Autodesk Inventor part; units mm, degrees
ref_plane "Arbeitsebene1" through (14, 0, 0) normal (1, 0, 0) x (0, 1, 0)
ref_plane "XZ Plane" through (0, 0, 0) normal (0, 1, 0) x (-1, 0, 0)
ref_plane "XY Plane" through (0, 0, 0) normal (0, 0, 1) x (1, 0, 0)
sketch "Skizze1" plane through (0, 0, 0) normal (0, 0, 1) x (1, 0, 0)
  line L0 (0, 20) -> (28, 20)
  line L1 (28, 20) -> (28, 0)
  line L2 (28, 0) -> (0, 0)
  line L3 (0, 0) -> (0, 20)
  dimension "d0" = 28
  dimension "d1" = 20
extrude "Extrusion1" add sketch "Skizze1" along normal blind 3
sketch "Skizze2" plane through (0, 0, 3) normal (0, 0, 1) x (1, 0, 0)
  line L0 (0, 20) -> (0, 0)
  line L1 (0, 10) -> (28.5763, 10) construction
  line L2 (28, 0) -> (28, 20)
  point P0 (3, 17)
  point P1 (3, 3)
  point P2 (25, 17)
  point P3 (25, 3)
  dimension "d4" = 14
  dimension "d5" = 3
  dimension "d14" = 3
hole "Bohrung1" at (3, 17, 3) at (3, 3, 3) at (25, 3, 3) at (25, 17, 3) direction (0, 0, -1) diameter 1.4 end through all countersink diameter 3 countersink angle 90
ref_plane "Arbeitsebene1" through (14, 0, 0) normal (1, 0, 0) x (0, 1, 0)
properties part number "Zylinderkopf" material "Stahl, galvanisiert"
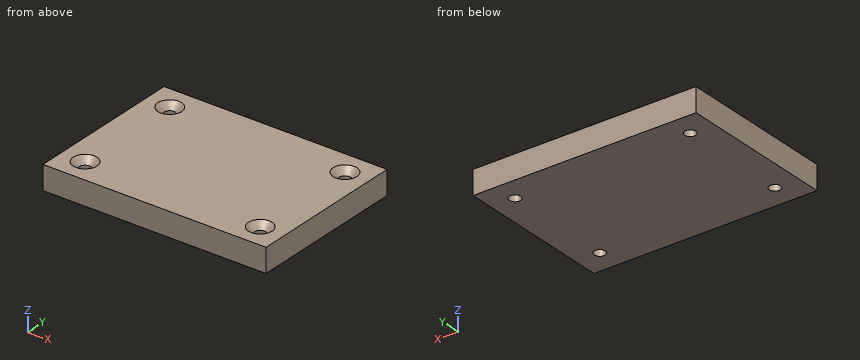
Here's how the part is built. I have some questions about the finished solid (model axes, mm). Give positions to 0.01 mm unless a question says otherwise; leave off trailing zeros. Loops run counter-clockwise (first coordinate to the right, second up) from the corner with the lowest first, then second, coordinate; pieces in that order, holes last. Notation, with made-up numbers: M -23.5,57 L -10.5,57 A5 cw -10.5,65 Z; hole C 41,36.25 d2. An arc over 180 degrees is marked long. Use one line per item in the form item = value. Start each with the question number.
Q1. If we section it at C-C (z = 2.65): Write out the boundary of the cut face in (x, y), then the cut area to 3 significant figures.
Q2. Will these pins go through, and if not, where does the flat tip stop? pin 1 Ø1.5 at (x, y) = (19.5, 8.5) entering from -Z; pin 2 Ø1.8 at (x, y) = (3, 17) entering from +Z.
Q3. If we section it at A-A (y = 3): Write out the boundary of the cut face in (x, z), then the cut area to 3 significant figures.
Q4. I need wall thicknesses on line 1 along Y through (x, z) = (25, 1.25); line 2 along X through (y, z) = (3, 1.1); line 3 along X through (y, z) = (3, 2.3). Which ranges of each line are inside material? Lowest first, please.
Q5. If we section it at B-B (x = 3): Write out the boundary of the cut face in (y, z).
Taken from the geometry:
q1.outline = M 0,0 L 28,0 L 28,20 L 0,20 Z; hole C 3,3 d2.3; hole C 3,17 d2.3; hole C 25,3 d2.3; hole C 25,17 d2.3
q1.area = 543 mm^2
q2.pin_1 = 0
q2.pin_2 = 2.4
q3.outline = M 0,0 L 2.3,0 L 2.3,2.2 L 1.5,3 L 0,3 Z; M 3.7,0 L 24.3,0 L 24.3,2.2 L 23.5,3 L 4.5,3 L 3.7,2.2 Z; M 25.7,0 L 28,0 L 28,3 L 26.5,3 L 25.7,2.2 Z
q3.area = 74.3 mm^2
q4.line_1 = 0 to 2.3, 3.7 to 16.3, 17.7 to 20
q4.line_2 = 0 to 2.3, 3.7 to 24.3, 25.7 to 28
q4.line_3 = 0 to 2.2, 3.8 to 24.2, 25.8 to 28
q5.outline = M 0,0 L 2.3,0 L 2.3,2.2 L 1.5,3 L 0,3 Z; M 3.7,0 L 16.3,0 L 16.3,2.2 L 15.5,3 L 4.5,3 L 3.7,2.2 Z; M 17.7,0 L 20,0 L 20,3 L 18.5,3 L 17.7,2.2 Z
